Could you check a few things on this drawing? It's one solid part, dimensions in mm from its lowest x, y, z. A direction names the side the tool comes from. Give positions to 0.01 mm unless a question says otherwise; leave off trailing zeros. Write each loop counter-clockwise with the first axis right and the second up, starting at its lowest first coordinate (ties: lowest second). Pieces come first, ordered by that corner, then holes. Notation, with made-up numbers: (4, -3.5) - (27, -3.5) arc R9 cw to (27, 7.5) - close; hole circle Ø2 at (9.25, 66.25). An arc over 180 degrees is marked (long way). One line per item, written item: value. Start each with the question number.
1) Please list where these lines run through material, in increasing order: L1, parallel to X at y = 3.5, z = 15; L2, parallel to X at y = 9.5, z = 20.5; L3, parallel to Y at x = 15, z = 19.25. Write a range as [from, to].
2) Imagine slicing it at B-B on x = 20. Write out the boundary of the cut face in (y, z).
3) Imagine slicing it at A-A on y = 11.5. Write out the boundary of the cut face in (x, z), plus the area to 3 significant figures.
4) On a 3-axis mill with a long thin cutter (end or side, diameter ignored), from which of +Z, -Z, +X, -X, +Y, -Y can I reach the whole of each face in a straight line? I mean the marked faces 1, 2 and 3. Say none if no direction works.
5) I'm going to push flat-ended pins straight in: P1, Ø3, axis at y = 25.5, z = 5, coming from the -X side; P2, Ø2, axis at x = 49.5, z = 7, coming from the -Y side; P3, Ø5, axis at x = 19, z = 13.5, coming from the +Y side. Where does each tip first touch, or does it pass through?
6) We'd pull the mould along X, two halves only. Please class the marked faces 4, 5 and 6: +X half, -X half, draft (parallel to the pull), parting line (faces both ways), or undercut.
7) Imagine slicing it at C-C on z = 15. Write out the boundary of the cut face in (x, y).
8) Imagine slicing it at D-D on z = 21. Write out the boundary of the cut face in (x, y).
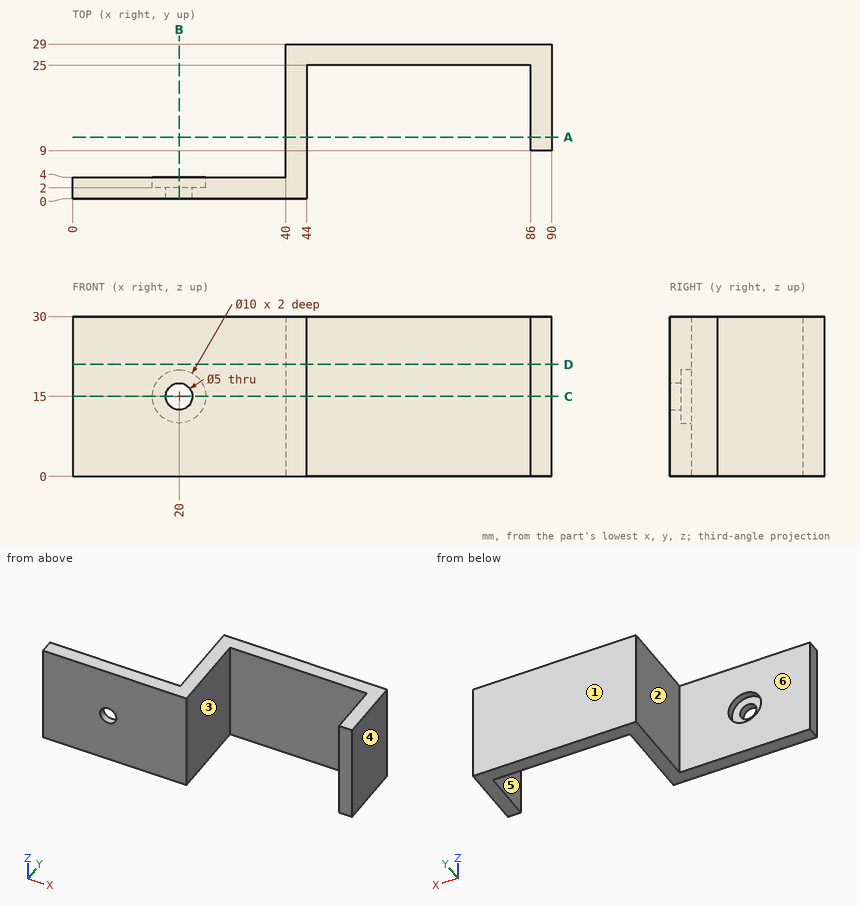
Numbers:
1. L1: [0, 15], [25, 44]
1. L2: [40, 44], [86, 90]
1. L3: [0, 4]
2. outline: (0, 0) - (4, 0) - (4, 10) - (2, 10) - (2, 12.5) - (0, 12.5) - close; (0, 17.5) - (2, 17.5) - (2, 20) - (4, 20) - (4, 30) - (0, 30) - close
3. outline: (40, 0) - (44, 0) - (44, 30) - (40, 30) - close; (86, 0) - (90, 0) - (90, 30) - (86, 30) - close
3. area: 240 mm^2
4. face 1: +Z, -Z, +X, -X, +Y
4. face 2: +Z, -Z, -X, +Y
4. face 3: +Z, -Z, -Y
5. P1: x = 40
5. P2: y = 25
5. P3: y = 2
6. face 4: +X half
6. face 5: undercut
6. face 6: draft
7. outline: (0, 0) - (17.5, 0) - (17.5, 2) - (15, 2) - (15, 4) - (0, 4) - close; (22.5, 0) - (44, 0) - (44, 25) - (86, 25) - (86, 9) - (90, 9) - (90, 29) - (40, 29) - (40, 4) - (25, 4) - (25, 2) - (22.5, 2) - close
8. outline: (0, 0) - (44, 0) - (44, 25) - (86, 25) - (86, 9) - (90, 9) - (90, 29) - (40, 29) - (40, 4) - (0, 4) - close
